from build123d import *

# Parameters (mm, degrees)
EXTRUDE_THIN1_DEPTH = 430
SKETCH2_R           = 2.1
CUT_EXTRUDE1_DEPTH  = 10
SKETCH3_W           = 27.877816903
SKETCH3_H           = 42.526750181
CUT_EXTRUDE2_DEPTH  = 10


with BuildPart() as part:
    # Sketch1 → Extrude-Thin1 (new body)
    with BuildSketch(Plane(origin=(0, 0, 0), x_dir=(1, 0, 0), z_dir=(0, 1, 0))):
        Polygon((-10.945454545, 0), (-10.945454545, 7.7), (6.054545455, 7.7), (6.054545455, 0), (5.054545455, 0), (5.054545455, 6.7), (-9.945454545, 6.7), (-9.945454545, 0), align=None)
    extrude(amount=EXTRUDE_THIN1_DEPTH)

    # Sketch2 → Cut-Extrude1 (cut)
    with BuildSketch(Plane.XY.offset(-6.7)):
        with Locations((-2.445454545, 390)):
            Circle(SKETCH2_R)
        with Locations(Location((-2.445454545, 40, 0), (0, 0, 180))):
            Circle(SKETCH2_R)
    extrude(amount=-CUT_EXTRUDE1_DEPTH, mode=Mode.SUBTRACT)

    # Sketch3 → Cut-Extrude2 (cut)
    with BuildSketch(Plane.XY):
        with Locations((-4.854182527, 416.263375091)):
            Rectangle(SKETCH3_W, SKETCH3_H)
    extrude(amount=-CUT_EXTRUDE2_DEPTH, mode=Mode.SUBTRACT)


solid = part.part
Could you check a few things on this model? Use its own coordinates, in mm. A direction names the side the tool comes from. Give positions to 0.01 mm unless a question says otherwise; leave off trailing zeros. Write each loop counter-clockwise with the first axis right and the second up, starting at its lowest first coordinate (ties: lowest second). Pieces come first, ordered by that corner, then holes. Notation, with made-up numbers: (-2, -32) -> (14, -32) arc R10 ccw to (14, -20) -> close; hole circle Ø9 at (-38, 85.5). An arc over 180 degrees is marked (long way). Write each question's results on one line, items separated by ' | '. Start each with the question number.
Q1. Suppose I cut it at B-B, the plane y = 155. List the corners of the cut face in (x, z) for me, and give its area (3 significant figures).
Q2. Which directions (+Z, -Z, +X, -X, +Y, -Y) give clear straight access to the entire face, cutting with the end or side of a thin tool? Please do faces 1 (the face through (-10.945, 195, -4)), 2 (the face through (-2, 195, -6.7)).
Q3. We'd pull the mould along X, two halves only. Please class faces 3 (the face through (-2, 395, -7)), 4 (the face through (-9.945, 195, -3)), 5 (the face through (6.055, 195, -4)): +X half, -X half, draft (parallel to the pull), parting line (faces both ways), or undercut.
Q4. I need wall thicknesses on probe 1 along X at (y, z) = (40, -6.95); probe 2 along X at (y, z) = (30, -1); probe 3 along Y at (x, z) = (-0.75, -7.5). Which ranges of each line are inside material? Lowest first, please.
Q5. Suppose I cut it at A-A, the plane z = -2.75. List the corners of the cut face in (x, y) for me, and give its area (3 significant figures).
Q6. I'm going to push a flat-ended pin straight in: pin 1 Ø5.5 at (x, y) = (-2.45, 40) entering from +Z. Where does the tip first touch, or does it pass through?
Outcome:
1) outline: (-10.95, -7.7) -> (6.05, -7.7) -> (6.05, 0) -> (5.05, 0) -> (5.05, -6.7) -> (-9.95, -6.7) -> (-9.95, 0) -> (-10.95, 0) -> close | area: 30.4 mm2
2) face 1: +Z, -Z, -X, +Y, -Y | face 2: +Z, +Y, -Y
3) face 3: draft | face 4: undercut | face 5: +X half
4) probe 1: -10.95 to -4.55, -0.35 to 6.05 | probe 2: -10.95 to -9.95, 5.05 to 6.05 | probe 3: 0 to 38.76, 41.24 to 388.76, 391.24 to 395
5) outline: (-10.95, 0) -> (-9.95, 0) -> (-9.95, 395) -> (-10.95, 395) -> close; (5.05, 0) -> (6.05, 0) -> (6.05, 395) -> (5.05, 395) -> close | area: 790 mm2
6) pin 1: z = -6.7
